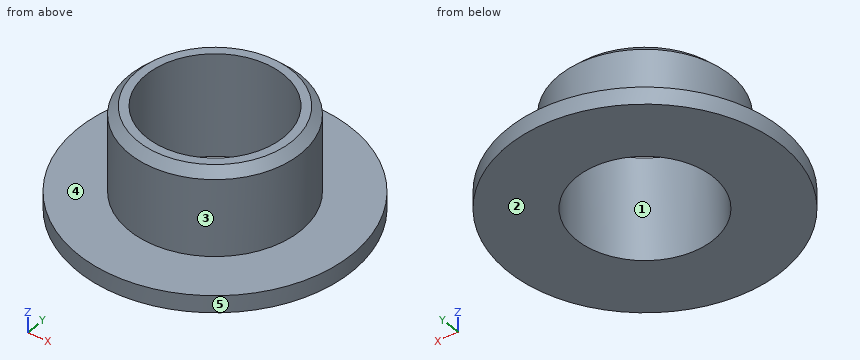
Autodesk Inventor part; units mm, degrees
ref_plane "YZ Plane" through (0, 0, 0) normal (1, 0, 0) x (0, 1, 0)
ref_plane "XZ Plane" through (0, 0, 0) normal (0, 1, 0) x (-1, 0, 0)
ref_plane "XY Plane" through (0, 0, 0) normal (0, 0, 1) x (1, 0, 0)
sketch "スケッチ1" plane through (0, 0, 0) normal (0, 0, 1) x (1, 0, 0)
  circle A0 centre (0, 0) radius 4
  circle A1 centre (0, 0) radius 8
  dimension "d0" = 8
  dimension "d1" = 16
extrude "押し出し1" add sketch "スケッチ1" along normal blind 1
sketch "スケッチ2" plane through (0, 0, 1) normal (0, 0, 1) x (1, 0, 0)
  circle A0 centre (0, 0) radius 5
  circle A1 centre (0, 0) radius 8
  circle A2 centre (0, 0) radius 4
  dimension "d4" = 10
extrude "押し出し2" add sketch "スケッチ2" along normal blind 5 contours A0
chamfer "面取り1" distance 0.5 angle 45 1 edges at (-5, 0, 6)
properties part number "オイレスw3f10-8a" material "アセタール樹脂、黒"
The model under review builds one solid part; all positions refer to its coordinate system, in mm. Face numbers are marked on the shaded views. A direction names the side the tool comes from. Coordinates: 2 decimals unless noted, no trailing zeros. Loops run counter-clockwise (first coordinate to the right, second up) from the corner with the lowest first, then second, coordinate; pieces in that order, holes last. Notation, with made-up numbers: (-40, 8.25) -> (-3, 8.25) arc R23 cw to (-3, 45.25) -> close; hole circle Ø9 at (20.25, 28). An arc over 180 degrees is marked (long way). Answer as CSV lines item,"result".
Item 1: Take a section at D-D, the plane x = -6.5. State the section outline as (y, z) points.
Results below:
outline,"(-4.66, 0) -> (4.66, 0) -> (4.66, 1) -> (-4.66, 1) -> close"
Item 2: Machinability: for the marked faces 4 and 5, which of the approach directions +Z, -Z, +X, -X, +Y, -Y give a long, thin tool a straight path to every point of the face, cutting with its end or side? Answer none if there is none.
Results below:
face 4,"+Z"
face 5,"+Z, -Z"
Item 3: Take a section at C-C, the plane z = 4. State the section outline as (x, y) points.
Results below:
outline,"circle Ø10 at (0, 0); hole circle Ø8 at (0, 0)"
Item 4: For L1, parallel to Y at x = 0, z = 4.05; L2, parallel to X at y = 1.25, z = 3.85; L3, parallel to Z at x = 1.5, y = -5.75, list the stretches that pass through material, from the lowest coordinate up.
Results below:
L1,"y = -5 to -4, 4 to 5"
L2,"x = -4.84 to -3.8, 3.8 to 4.84"
L3,"z = 0 to 1"
Item 5: Draft analysis for pull direction Y (two halves, no side actions). For the marked faces 1, 2 and 3, state which applies: +Y half, -Y half, draft (parallel to the pull), parting line (faces both ways), or undercut.
Results below:
face 1,"undercut"
face 2,"draft"
face 3,"parting line"
Item 6: Insertion check: pin 1 (4 mm diameter, centred on x = -6.5, y = -5.5, fed in from +Z); pin 2 (8 mm diameter, centred on x = -1, y = 3.5, fed in from +Z). Each pin has a flat end and moves straight along its axis. Give the tip position at first contact, or say it passes through.
Results below:
pin 1,"stops at z = 1"
pin 2,"stops at z = 6"
Item 7: Take a section at A-A, the plane x = 0. State the section outline as (y, z) points.
Results below:
outline,"(-8, 0) -> (-4, 0) -> (-4, 6) -> (-4.5, 6) -> (-5, 5.5) -> (-5, 1) -> (-8, 1) -> close; (4, 0) -> (8, 0) -> (8, 1) -> (5, 1) -> (5, 5.5) -> (4.5, 6) -> (4, 6) -> close"
